from build123d import *

# Parameters (mm, degrees)
F0_W      = 177.8
F0_H      = 260.35
F1_DEPTH  = 25.4
F2_W      = 10.16
F2_H      = 5.588
F2_W_2    = 12.7
F2_H_2    = 6.604
F3_DEPTH  = 25.401
F4_W      = 145.796
F4_H      = 110.49
F5_DEPTH  = 8.466667
F6_W      = 41.43375
F6_H      = 12.8016
F7_DEPTH  = 6.35
F6_W_2    = 43.02125
F6_H_2    = 9.525
F8_DEPTH  = 4.445
F6_W_3    = 15.39875
F6_W_4    = 13.81125
F9_DEPTH  = 10.16
F10_W     = 101.6
F10_H     = 25.4
F11_DEPTH = 11.43


with BuildPart() as f1:
    # F0 (on Top) → F1 (new body)
    with BuildSketch(Plane.XY):
        Rectangle(F0_W, F0_H)
    extrude(amount=F1_DEPTH)

    # F2 (on face) → F3 (cut, through all)
    with BuildSketch(Plane.XY.offset(25.4)):
        with Locations((0, 130.175)):
            Rectangle(F2_W, F2_H)
        with Locations((0, -130.175)):
            Rectangle(F2_W_2, F2_H_2)
    extrude(amount=-F3_DEPTH, mode=Mode.SUBTRACT)

    # F4 (on face) → F5 (cut)
    with BuildSketch(Plane.XY.offset(25.4)):
        with Locations((0, 62.23)):
            Rectangle(F4_W, F4_H)
    extrude(amount=-F5_DEPTH, mode=Mode.SUBTRACT)

    # F6 (on face) → F7 (cut)
    with BuildSketch(Plane.XY.offset(25.4)):
        with Locations((-51.355625, -56.515)):
            Rectangle(F6_W, F6_H)
        with Locations((51.355625, -56.515)):
            Rectangle(F6_W, F6_H)
        with Locations((51.355625, -34.925)):
            Rectangle(F6_W, F6_H)
    extrude(amount=-F7_DEPTH, mode=Mode.SUBTRACT)

    # F6 (on face) → F8 (cut)
    with BuildSketch(Plane.XY.offset(25.4)):
        with Locations((-52.149375, -34.925)):
            Rectangle(F6_W_2, F6_H_2)
        with Locations((-52.149375, -78.105)):
            Rectangle(F6_W_2, F6_H_2)
        with Locations((-52.149375, -99.695)):
            Rectangle(F6_W_2, F6_H_2)
        with Locations((52.149375, -78.105)):
            Rectangle(F6_W_2, F6_H_2)
        with Locations((52.149375, -99.695)):
            Rectangle(F6_W_2, F6_H_2)
    extrude(amount=-F8_DEPTH, mode=Mode.SUBTRACT)

    # F6 (on face) → F9 (cut)
    with BuildSketch(Plane.XY.offset(25.4)):
        Polygon((-15.24, -30.1625), (-15.24, -39.6875), (-30.63875, -39.6875), (-30.63875, -50.1142), (-16.8275, -50.1142), (-16.8275, -62.9158), (-30.63875, -62.9158), (-30.63875, -73.3425), (-15.24, -73.3425), (-15.24, -82.8675), (-30.63875, -82.8675), (-30.63875, -94.9325), (-15.24, -94.9325), (-15.24, -104.4575), (-30.63875, -104.4575), (-30.63875, -113.3475), (30.63875, -113.3475), (30.63875, -104.4575), (15.24, -104.4575), (15.24, -94.9325), (30.63875, -94.9325), (30.63875, -82.8675), (15.24, -82.8675), (15.24, -73.3425), (30.63875, -73.3425), (30.63875, -62.9158), (16.8275, -62.9158), (16.8275, -50.1142), (30.63875, -50.1142), (30.63875, -41.3258), (16.8275, -41.3258), (16.8275, -28.5242), (30.63875, -28.5242), (30.63875, -19.6342), (-30.63875, -19.6342), (-30.63875, -30.1625), align=None)
        with Locations((-22.939375, -34.925)):
            Rectangle(F6_W_3, F6_H_2)
        with Locations((-23.733125, -56.515)):
            Rectangle(F6_W_4, F6_H)
        with Locations((-22.939375, -78.105)):
            Rectangle(F6_W_3, F6_H_2)
        with Locations((-22.939375, -99.695)):
            Rectangle(F6_W_3, F6_H_2)
        with Locations((22.939375, -99.695)):
            Rectangle(F6_W_3, F6_H_2)
        with Locations((22.939375, -78.105)):
            Rectangle(F6_W_3, F6_H_2)
        with Locations((23.733125, -56.515)):
            Rectangle(F6_W_4, F6_H)
        with Locations((23.733125, -34.925)):
            Rectangle(F6_W_4, F6_H)
    extrude(amount=-F9_DEPTH, mode=Mode.SUBTRACT)

    # F10 (on face) → F11 (cut)
    with BuildSketch(Plane(origin=(0, 0, 0), x_dir=(1, 0, 0), z_dir=(0, 0, -1))):
        with Locations((0, 41.275)):
            Rectangle(F10_W, F10_H)
        with Locations((0, -92.075)):
            Rectangle(F10_W, F10_H)
    extrude(amount=-F11_DEPTH, mode=Mode.SUBTRACT)


solid = f1.part
Geometry check sheet. Reference: the model listing, model coordinates, mm. A direction names the side the tool comes from. Give positions to 0.01 mm unless a question says otherwise; leave off trailing zeros. Write each loop counter-clockwise with the first axis right and the second up, starting at its lowest first coordinate (ties: lowest second). Pieces come first, ordered by that corner, then holes. Notation, with made-up numbers: M -12.5,2 L 31.5,2 A21 cw 31.5,32 Z; hole C -30,28.25 d5. An arc over 180 degrees is marked long. Answer as CSV lines item,"result". Start each with the question number.
Q1. Go/stop test with flat-tipped pins: pin 1 (1 mm diameter, centred on x = -3.5, z = 17, fed in from -Y); pin 2 (1.5 mm diameter, centred on x = 21, y = -37.5, fed in from +Z); pin 3 (3 mm diameter, centred on x = -51, y = -37, fed in from +Z) (3 decimals). Record where each tip stops, or that it passes through.
Q2. Section check A-A, the plane z = 8.75. Record the cut outline in (x, y) (3 decimals).
Q3. Tool access check on faces 1 (the face through (-48, 130.175, 13)), 2 (the face through (30.639, -67, 19)), 3 (the face through (-1, -28.575, 6)). Record the directions out of +Z, -Z, +X, -X, +Y, -Y that give a thin tool (end or side, any length) a straight path to the whole face; none if there is none.
Q4. Release check for a two-part mould opening along Y. For faces 4 (the face through (51, -28.524, 22)), 5 (the face through (-1, 2, 0)), 6 (the face through (47, -130.175, 13)) record: pulls with the +Y half, pulls with the -Y half, needs draft (parallel to the pull), parting line crosses it, or undercut.
Q5. Material ranges on L1, parallel to Y at x = 6.5, z = 21 (1 decimal); L2, parallel to Y at x = 27.5, z = 6.5 (3 decimals); L3, parallel to Y at x = -73, z = 21 (1 decimal), recorded low to high.
Q6. Section check C-C, the plane y = -47. Record the cut outline in (x, z).
Geometry says:
1,pin 1,"y = -126.87"
1,pin 2,"z = 15.24"
1,pin 3,"z = 20.955"
2,outline,"M -88.9,-130.175 L -6.35,-130.175 L -6.35,-126.873 L 6.35,-126.873 L 6.35,-130.175 L 88.9,-130.175 L 88.9,130.175 L 5.08,130.175 L 5.08,127.381 L -5.08,127.381 L -5.08,130.175 L -88.9,130.175 Z; hole M -50.8,-53.975 L 50.8,-53.975 L 50.8,-28.575 L -50.8,-28.575 Z; hole M -50.8,79.375 L 50.8,79.375 L 50.8,104.775 L -50.8,104.775 Z"
3,face 1,"+Z, -Z, +X, -X, +Y"
3,face 2,"+Z"
3,face 3,"-Z"
4,face 4,"undercut"
4,face 5,"needs draft"
4,face 6,"pulls with the -Y half"
5,L1,"-130.2 to -113.3, -19.6 to 7, 117.5 to 130.2"
5,L2,"-130.175 to -53.975, -28.575 to 79.375, 104.775 to 130.175"
5,L3,"-130.2 to -104.5, -94.9 to -82.9, -73.3 to -39.7, -30.2 to 130.2"
6,outline,"M -88.9,0 L -50.8,0 L -50.8,11.43 L 50.8,11.43 L 50.8,0 L 88.9,0 L 88.9,25.4 L 30.64,25.4 L 30.64,15.24 L -30.64,15.24 L -30.64,25.4 L -88.9,25.4 Z"
